Can you work these out from the model? Positions are in its coordinate system, mm. A direction names the side the tool comes from. Coordinates: 2 decimals unless noted, no trailing zeros. Write each loop counter-clockwise with the first axis right and the second up, starting at its lowest first coordinate (ties: lowest second). Pieces come first, ordered by that corner, then holes. Notation, with made-up numbers: (85.5, -1.5) -> (121.5, -1.5) arc R20 ccw to (121.5, 17.5) -> close; hole circle Ø3 at (-15.75, 69). An arc over 180 degrees is marked (long way). Use one line per item in the form item = value.
```python
from build123d import *

# Parameters (mm, degrees)
ARA_D_ZLEM_R                = 50
BASE_DEPTH                  = 5
Y_KSEKLIK_EKSTR_ZYON2_DEPTH = 40
IZIM2_R                     = 2
BANANA_SLOTLAR_DEPTH        = 82.240384046
IZIM3_R                     = 2
IZIM3_R_2                   = 5.05
KES_EKSTR_ZYON1_DEPTH       = 5
IZIM3_2_R                   = 2
KES_EKSTR_ZYON2_DEPTH       = 82.240384046
IZIM5_R                     = 3.6
KES_EKSTR_ZYON3_DEPTH       = 79.89866919


with BuildPart() as part:
    # ara d_zlem → base (new body)
    with BuildSketch(Plane(origin=(0, 0, 0), x_dir=(1, 0, 0), z_dir=(0, 1, 0))):
        with Locations(Location((0, 0, 0), (0, 0, 270))):
            Circle(ARA_D_ZLEM_R)
    extrude(amount=BASE_DEPTH)

    # izim1_3 → Y_kseklik-Ekstr_zyon2 (add)
    with BuildSketch(Plane(origin=(0, 0, 0), x_dir=(1, 0, 0), z_dir=(0, 1, 0))):
        with BuildLine():
            ThreePointArc((28.7, 40.942764929), (0, 50), (-28.7, 40.942764929))
            Line((-28.7, 40.942764929), (-28.7, -40.942764929))
            ThreePointArc((-28.7, -40.942764929), (0, -50), (28.7, -40.942764929))
            Line((28.7, -40.942764929), (28.7, 40.942764929))
        make_face()
    extrude(amount=Y_KSEKLIK_EKSTR_ZYON2_DEPTH)

    # izim2 → banana slotlar (cut, through all)
    with BuildSketch(Plane(origin=(0, 40, 0), x_dir=(1, 0, 0), z_dir=(0, 1, 0))):
        with Locations(Location((-11.3, -24.942764929, 0), (0, 0, 270))):
            Circle(IZIM2_R)
        with Locations(Location((-11.3, -36.942764929, 0), (0, 0, 90))):
            Circle(IZIM2_R)
    extrude(amount=-BANANA_SLOTLAR_DEPTH, mode=Mode.SUBTRACT)

    # izim3 → Kes-Ekstr_zyon1 (cut)
    with BuildSketch(Plane.XZ):
        with Locations(Location((-29.69848481, 29.69848481, 0), (0, 0, 270))):
            Circle(IZIM3_R)
        with Locations(Location((29.69848481, 29.69848481, 0), (0, 0, 270))):
            Circle(IZIM3_R)
        with Locations(Location((29.69848481, -29.69848481, 0), (0, 0, 270))):
            Circle(IZIM3_R)
        with Locations(Location((-29.69848481, -29.69848481, 0), (0, 0, 270))):
            Circle(IZIM3_R)
        with Locations(Location((0, 0, 0), (0, 0, 270))):
            Circle(IZIM3_R_2)
    extrude(amount=-KES_EKSTR_ZYON1_DEPTH, mode=Mode.SUBTRACT)

    # izim3_2 → Kes-Ekstr_zyon2 (cut, through all)
    with BuildSketch(Plane.XZ):
        with Locations(Location((-29.69848481, 29.69848481, 0), (0, 0, 270))):
            Circle(IZIM3_2_R)
        with Locations(Location((-29.69848481, -29.69848481, 0), (0, 0, 270))):
            Circle(IZIM3_2_R)
        with Locations(Location((29.69848481, -29.69848481, 0), (0, 0, 270))):
            Circle(IZIM3_2_R)
        with Locations(Location((29.69848481, 29.69848481, 0), (0, 0, 270))):
            Circle(IZIM3_2_R)
    extrude(amount=-KES_EKSTR_ZYON2_DEPTH, mode=Mode.SUBTRACT)

    # izim5 → Kes-Ekstr_zyon3 (cut, through all)
    with BuildSketch(Plane(origin=(0, 5, 0), x_dir=(1, 0, 0), z_dir=(0, 1, 0))):
        with Locations((29.69848481, -29.69848481)):
            Circle(IZIM5_R)
        with Locations((-29.69848481, -29.69848481)):
            Circle(IZIM5_R)
        with Locations((-29.69848481, 29.69848481)):
            Circle(IZIM5_R)
        with Locations((29.69848481, 29.69848481)):
            Circle(IZIM5_R)
    extrude(amount=KES_EKSTR_ZYON3_DEPTH, mode=Mode.SUBTRACT)


solid = part.part
```
Q1. Suppose I cut it at A-A (y = 16.5). Write out the boundary of the cut face in (x, z), then the cut area to 3 significant figures.
Return value:
outline = (-28.7, -40.94) arc R50 ccw to (28.7, -40.94) -> (28.7, -33.16) arc R3.6 cw to (28.7, -26.24) -> (28.7, 26.24) arc R3.6 cw to (28.7, 33.16) -> (28.7, 40.94) arc R50 ccw to (-28.7, 40.94) -> (-28.7, 33.16) arc R3.6 cw to (-28.7, 26.24) -> (-28.7, -26.24) arc R3.6 cw to (-28.7, -33.16) -> close; hole circle Ø4 at (-11.3, 24.94); hole circle Ø4 at (-11.3, 36.94)
area = 5,330 mm2
Q2. If I drill on line 1 (X direction, y = 32, z = 34); line 2 (Y direction, x = -36.5, z = -19.5); line 3 (Z direction, x = -19, y = 11), over which ranges is the centre line in solid material (lowest first)? Write a range as from..to.
Return value:
line_1 = -28.7..28.7
line_2 = 0..5
line_3 = -46.25..46.25
Q3. Will these pins go through, and if not, where does the flat tip stop? pin 1 (1.5 mm diameter, centred on y = 30.5, z = 26, fed in from +X); pin 2 (1.5 mm diameter, centred on y = 12, z = 9.5, fed in from -X); pin 3 (3.5 mm diameter, centred on x = 29.7, z = 29.7, fed in from -Y); pin 4 (5 mm diameter, centred on x = -29.7, z = 29.7, fed in from +Y).
Return value:
pin_1 = 28.7
pin_2 = -28.7
pin_3 = through
pin_4 = 5
Q4. Thinking about a two-plate mould opening in Z: for faces 1 (the flat face through (28.7, 22, 37)), 2 (the cylindrical face through (26.1, 22.3, -29.8)), 3 (the cylindrical face through (-10.534, 20.28, 35.095)), which applies, released by +Z, released by -Z, zero draft, split by the parting line, or undercut?
Return value:
face_1 = zero draft
face_2 = undercut
face_3 = undercut
Q5. Suppose I cut it at B-B (z = 0). Write out the boundary of the cut face in (x, y).
Return value:
outline = (-50, 0) -> (-5.05, 0) -> (-5.05, 5) -> (5.05, 5) -> (5.05, 0) -> (50, 0) -> (50, 5) -> (28.7, 5) -> (28.7, 40) -> (-28.7, 40) -> (-28.7, 5) -> (-50, 5) -> close
Q6. For faces 4 (the flat face through (-28.7, 22, 0)), 5 (the flat face through (28.7, 22, -37)), 6 (the flat face through (0, 5, 0)), 7 (the cylindrical face through (26.1, 22.3, 29.6)), which set-ups out of +Z, -Z, +X, -X, +Y, -Y let a thin tool reach every point of the face, with its end or its side?
Return value:
face_4 = +Z, -Z, -X, +Y
face_5 = +Z, -Z, +X, +Y
face_6 = -Y
face_7 = +X, +Y
Q7. Suppose I cut it at D-D (x = 24.5). Write out the boundary of the cut face in (y, z).
Return value:
outline = (0, -43.59) -> (40, -43.59) -> (40, 43.59) -> (0, 43.59) -> close
